Can you work these out from the model? Positions are in its coordinate system, mm. A direction names the side the tool comes from. Give positions to 0.01 mm unless a question says otherwise; leave off trailing zeros. Loops run counter-clockwise (first coordinate to the right, second up) from the corner with the lowest first, then second, coordinate; pieces in that order, holes last. Notation, with made-up numbers: (-13.75, 36.25) - (18.25, 36.25) arc R29 ccw to (18.25, 72.25) - close; hole circle Ø10 at (-19, 76). An arc over 180 degrees is marked (long way). Write item = value, one per line.
from build123d import *

# Parameters (mm, degrees)
F0_W     = 25.4
F0_H     = 3.4750678155
F1_DEPTH = 5.08
F0_W_2   = 12.7
F0_H_2   = 15.7407342222
F2_DEPTH = 7.62
F0_H_3   = 4.1556985352
F0_H_4   = 3.3092657778
F3_DEPTH = 12.7


with BuildPart() as f1:
    # F0 (on Top) → F1 (new body)
    with BuildSketch(Plane.XY):
        Polygon((-36.596847949, 53.1499683857), (-36.596847949, -73.2352957129), (-30.246847949, -73.2352957129), (-30.246847949, -57.4945614907), (-30.246847949, -53.3388629556), (-30.246847949, -19.8709424585), (-30.246847949, -15.9986205399), (-30.246847949, 50.9313653009), (-23.5789932814, 59.3087746812), (-17.546847949, 51.7300625752), (-17.546847949, -15.9986205399), (-17.546847949, -19.8709424585), (-17.546847949, -53.3388629556), (-17.546847949, -57.4945614907), (-17.546847949, -73.2352957129), (-11.196847949, -73.2352957129), (-11.196847949, 53.94866566), (-23.5789932814, 69.5054385093), align=None)
        Polygon((-36.596847949, -73.2352957129), (-36.596847949, -79.4194936752), (-11.196847949, -79.4194936752), (-11.196847949, -73.2352957129), (-17.546847949, -73.2352957129), (-17.546847949, -76.5445614907), (-30.246847949, -76.5445614907), (-30.246847949, -73.2352957129), align=None)
        with Locations((-23.896847949, -81.157027583)):
            Rectangle(F0_W, F0_H)
    extrude(amount=F1_DEPTH)

    # F0 (on Top) → F2 (join)
    with BuildSketch(Plane.XY):
        with Locations((-23.896847949, -65.3649286018)):
            Rectangle(F0_W_2, F0_H_2)
        Polygon((-30.246847949, -19.8709424585), (-30.246847949, -53.3388629556), (-17.546847949, -53.3388629556), (-17.546847949, -19.8709424585), (-17.546847949, -15.9986205399), (-17.546847949, 51.7300625752), (-23.5789932814, 59.3087746812), (-30.246847949, 50.9313653009), (-30.246847949, -15.9986205399), align=None)
    extrude(amount=F2_DEPTH)

    # F0 (on Top) → F3 (join)
    with BuildSketch(Plane.XY):
        with Locations((-23.896847949, -55.4167122231)):
            Rectangle(F0_W_2, F0_H_3)
        with Locations((-23.896847949, -74.8899286018)):
            Rectangle(F0_W_2, F0_H_4)
    extrude(amount=F3_DEPTH)


solid = f1.part
Q1. Imagine slicing it at D-D, the plane z = 1.5. Write out the boundary of the cut face in (x, y), then the cut area to 3 significant figures.
Output:
outline = (-36.6, -82.89) - (-11.2, -82.89) - (-11.2, 53.95) - (-23.58, 69.51) - (-36.6, 53.15) - close
area = 3,670 mm2
Q2. I need wall thicknesses on L1, parallel to Y at x = -19.5, z = 12; L2, parallel to Z at x = -26, y = 62; L3, parallel to Z at x = -27.5, y = -41.5. Which ranges of each line are inside material? Lowest first, please.
Output:
L1 = -76.54 to -73.24, -57.49 to -53.34
L2 = 0 to 5.08
L3 = 0 to 7.62
Q3. Imagine slicing it at B-B, the plane y = -13.5. Write out the boundary of the cut face in (x, z).
Output:
outline = (-36.6, 0) - (-11.2, 0) - (-11.2, 5.08) - (-17.55, 5.08) - (-17.55, 7.62) - (-30.25, 7.62) - (-30.25, 5.08) - (-36.6, 5.08) - close
Q4. Which directions (+Z, -Z, +X, -X, +Y, -Y) give clear straight access to the entire face, cutting with the end or side of a thin tool? Please do faces 1 (the flat face through (-20.521, 55.466, 6.332)), 2 (the flat face through (-24, 4, 7.62)), 3 (the flat face through (-24, -73.235, 10)), 4 (the flat face through (-17.547, -28, 7)), 5 (the flat face through (-24, -76.545, 9)).
Output:
face_1 = +Z, +X, +Y
face_2 = +Z, +X, -X, +Y
face_3 = +Z, +X, -X
face_4 = +Z, +X, +Y, -Y
face_5 = +Z, +X, -X, -Y
Q5. Imagine slicing it at C-C, the plane x = -28. Write out the boundary of the cut face in (y, z).
Output:
outline = (-82.89, 0) - (63.95, 0) - (63.95, 5.08) - (53.75, 5.08) - (53.75, 7.62) - (-53.34, 7.62) - (-53.34, 12.7) - (-57.49, 12.7) - (-57.49, 7.62) - (-73.24, 7.62) - (-73.24, 12.7) - (-76.54, 12.7) - (-76.54, 5.08) - (-82.89, 5.08) - close
Q6. For pin 1 (5.5 mm diameter, centred on x = -24.5, z = 11, fed in from -Y); pin 2 (5 mm diameter, centred on x = -27, z = 6.5, fed in from -Y); pin 3 (2.5 mm diameter, centred on y = 6.5, z = 9, fed in from -X); pin 4 (6.5 mm diameter, centred on x = -23, y = 7.5, fed in from +Z), each with a flat end and sliding along its axis, tell me the tip position at first contact or that it passes through.
Output:
pin_1 = -76.54
pin_2 = -82.89
pin_3 = through
pin_4 = 7.62
Q7. Imagine slicing it at A-A, the plane z = 9. Write out the boundary of the cut face in (x, y), then the cut area to 3 significant figures.
Output:
outline = (-30.25, -76.54) - (-17.55, -76.54) - (-17.55, -73.24) - (-30.25, -73.24) - close; (-30.25, -57.49) - (-17.55, -57.49) - (-17.55, -53.34) - (-30.25, -53.34) - close
area = 94.8 mm2
Q8. We'd pull the mould along Y, two halves only. Please class faces 6 (the flat face through (-24, -57.495, 10)), 7 (the flat face through (-26.866, 55.179, 6.332)), 8 (the flat face through (-24, -82.895, 3)): released by +Y, released by -Y, zero draft, split by the parting line, or undercut.
Output:
face_6 = undercut
face_7 = released by +Y
face_8 = released by -Y
